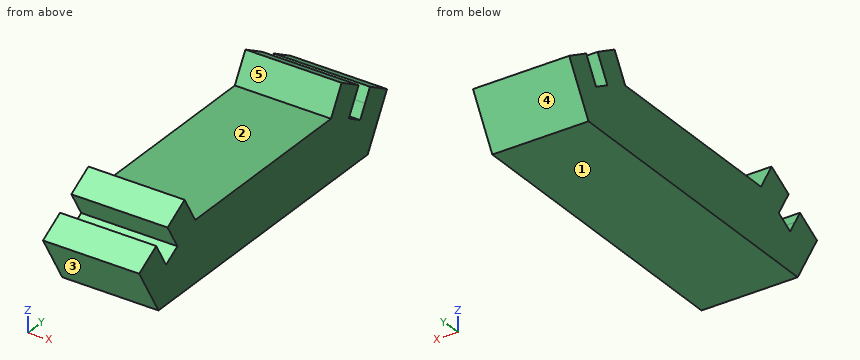
from build123d import *

# Parameters (mm, degrees)
EXTRUDE_1_DEPTH = 10


with BuildPart() as part:
    # Эскиз1 → Бобышка-Вытянуть1 (new body)
    with BuildSketch(Plane(origin=(0, 0, 0), x_dir=(0, 0, -1), z_dir=(1, 0, 0))):
        Polygon((-2.039845048, 21.046884737), (-4.637921259, 22.546884737), (-6.137921259, 19.948808526), (-3.338883154, 18.332783122), (-3.338883154, -2.399013647), (-6.137921259, -4.015039051), (-4.637921259, -6.613115263), (-2.039845048, -5.113115263), (-1.039845048, -6.84516607), (-2.338883154, -7.59516607), (-3.637921259, -8.34516607), (-2.137921259, -10.943242281), (2.960154952, -7.999866609), (2.960154952, 23.933636083), (-2.137921259, 26.877011756), (-3.637921259, 24.278935545), (-2.338883154, 23.528935545), (-1.039845048, 22.778935545), align=None)
    extrude(amount=EXTRUDE_1_DEPTH)


solid = part.part
Verification items for the finished model (mm, model axes). Face numbers are marked on the shaded views. A direction names the side the tool comes from. Round coordinates to 2 decimals unless told otherwise and drop trailing zeros. Loops run counter-clockwise (first coordinate to the right, second up) from the corner with the lowest first, then second, coordinate; pieces in that order, holes last. Notation, with made-up numbers: M 43.5,0 L 60.5,0 A11 ccw 60.5,5 Z; hole C -2.75,-34.5 d6. An arc over 180 degrees is marked long. Write each question's results on one line, items separated by ' | '.
1) Mould release check, pull along Y, two halves, no side actions. Record for the marked faces 1, 2 and 3: released by +Y, released by -Y, zero draft, split by the parting line, or undercut.
Checks:
face 1: zero draft | face 2: undercut | face 3: released by -Y
2) Section check D-D on z = -1.5. Record the boundary of the cut face in (x, y).
Checks:
outline: M 0,-8.84 L 10,-8.84 L 10,24.78 L 0,24.78 Z
3) Section check C-C on y = 4. Record the boundary of the cut face in (x, z), then the cut area to 3 significant figures.
Checks:
outline: M 0,-2.96 L 10,-2.96 L 10,3.34 L 0,3.34 Z | area: 63.0 mm2
4) Gauge pin test, flat ends, axial feed: P1, Ø4, axis at x = 5, z = 2.5, coming from the -Y side; P2, Ø5, axis at x = 6, z = -1, coming from the -Y side; P3, Ø4, axis at x = 5, y = 20, coming from the +Z side. Record the tip position at first contact, or that the pin passes through.
Checks:
P1: stops at y = -10.94 | P2: stops at y = -10.57 | P3: stops at z = 6.14
5) Section check B-B on z = 4.25. Record the boundary of the cut face in (x, y), then the cut area to 3 significant figures.
Checks:
outline: M 0,-6.39 L 10,-6.39 L 10,-2.93 L 0,-2.93 Z; M 0,18.86 L 10,18.86 L 10,22.32 L 0,22.32 Z | area: 69.3 mm2
6) Access from +Z, -Z, +X, -X, +Y, -Y to the whole of each face (thin tool, end or side, straight path). Record for the marked faces 4 and 5.
Checks:
face 4: -Z, +X, -X, +Y | face 5: +Z, +X, -X
7) Scan lines: L1, parallel to Y at x = 7.5, z = 2; L2, parallel to Z at x = 7.25, y = -2; L3, parallel to Y at x = 7, z = 1.25. Record each from-to range of solid material in increasing order. Write a range as from..to.
Checks:
L1: y = -10.86..-7.4, -5.18..21.12, 23.33..26.8 | L2: z = -2.96..3.34 | L3: y = -10.43..-6.97, -6.48..22.41, 22.9..26.36
8) Section check A-A on x = 2.25. Record the boundary of the cut face in (y, z), then the cut area to 3 significant figures.
Checks:
outline: M -10.94,2.14 L -8,-2.96 L 23.93,-2.96 L 26.88,2.14 L 24.28,3.64 L 22.78,1.04 L 21.05,2.04 L 22.55,4.64 L 19.95,6.14 L 18.33,3.34 L -2.4,3.34 L -4.02,6.14 L -6.61,4.64 L -5.11,2.04 L -6.85,1.04 L -8.35,3.64 Z | area: 227 mm2
